For this review, take the finished solid that the model builds, in its own axes (mm). A direction names the side the tool comes from. Round coordinates to 2 decimals unless told otherwise and drop trailing zeros. Loops run counter-clockwise (first coordinate to the right, second up) from the corner with the lowest first, then second, coordinate; pieces in that order, holes last.
1) Mouldability with a two-part tool opening along Y and no side actions: class faces 4 (the cylindrical face through (-1.216, 1.115, 1.479)), 5 (the flat face through (34, 47, 1)), 6 (the flat face through (5.5, 44, 2)) as pulls with the +Y half, pulls with the -Y half, needs draft (parallel to the pull), parting line crosses it, or undercut.
2) Insertion check: pin 1 (19.5 mm diameter, centred on x = 10, z = 19, fed in from -Y); pin 2 (1 mm diameter, centred on x = 30, y = 7, fed in from +Z); pin 3 (3.5 mm diameter, centred on x = 21, z = 2, fed in from +Y); pin 4 (2.5 mm diameter, centred on x = 1, z = 10, fed in from +Y). Each pin has a flat end and moves straight along its axis. Give the tip position at first contact, or say it passes through.
3) Tool access review of faces 1 (the flat face through (17, 37, 14)), 2 (the cylindrical face through (30.07, 46.4, 1.48)), 3 (the flat face through (17, 34, 14)): name each direction out of +Z, -Z, +X, -X, +Y, -Y from which nothing blocks a thin tool from reaching the whole face with its end or side.
4) Take a section at B-B (z = 10). State the section outline as (x, y) points, then the cut area to 3 significant figures.
5) Take a section at D-D (y = 0). State the section outline as (x, z) points, then the cut area to 3 significant figures.
6) Take a section at A-A (y = 44). State the section outline as (x, z) points.
7) Take a section at C-C (x = 34). State the section outline as (y, z) points, then the cut area to 3 significant figures.
8) Wall thickness on L1, parallel to Z at x = 34, y = 35; L2, parallel to X at y = 34.75, z = 10; L3, parallel to Y at x = 0, z = 2.25: over which ranges is each line inside the solid? List them lowest first.
```python
from build123d import *

# Parameters (mm, degrees)
SKETCH1_W           = 41
SKETCH1_H           = 50
SKETCH1_R           = 1.65
BOSS_EXTRUDE1_DEPTH = 3
SKETCH2_W           = 41
SKETCH2_H           = 3
BOSS_EXTRUDE2_DEPTH = 30
SKETCH3_R           = 1.65
SKETCH3_R_2         = 7.5
CUT_EXTRUDE1_DEPTH  = 35
SKETCH4_W           = 24
SKETCH4_H           = 6
CUT_EXTRUDE2_DEPTH  = 10
FILLET2_R           = 2


with BuildPart() as part:
    # Sketch1 → Boss-Extrude1 (new body)
    with BuildSketch(Plane.XY):
        with Locations((17.5, 22)):
            Rectangle(SKETCH1_W, SKETCH1_H)
        with Locations((0, 44)):
            Circle(SKETCH1_R, mode=Mode.SUBTRACT)
        with Locations((35, 44)):
            Circle(SKETCH1_R, mode=Mode.SUBTRACT)
        with Locations((35, 0)):
            Circle(SKETCH1_R, mode=Mode.SUBTRACT)
        Circle(SKETCH1_R, mode=Mode.SUBTRACT)
    extrude(amount=BOSS_EXTRUDE1_DEPTH)

    # Sketch2 → Boss-Extrude2 (add)
    with BuildSketch(Plane.XY.offset(3)):
        with Locations((17.5, 35.5)):
            Rectangle(SKETCH2_W, SKETCH2_H)
    extrude(amount=BOSS_EXTRUDE2_DEPTH)

    # Sketch3 → Cut-Extrude1 (cut)
    with BuildSketch(Plane(origin=(0, 37, 0), x_dir=(1, 0, 0), z_dir=(0, 1, 0))):
        with Locations((34, -28)):
            Circle(SKETCH3_R)
        with Locations((34, -10)):
            Circle(SKETCH3_R)
        with Locations((1, -10)):
            Circle(SKETCH3_R)
        with Locations((1, -28)):
            Circle(SKETCH3_R)
        with Locations((10, -19)):
            Circle(SKETCH3_R_2)
    extrude(amount=-CUT_EXTRUDE1_DEPTH, mode=Mode.SUBTRACT)

    # Sketch4 → Cut-Extrude2 (cut)
    with BuildSketch(Plane.XY.offset(3)):
        with Locations((17.5, 44)):
            Rectangle(SKETCH4_W, SKETCH4_H)
    extrude(amount=-CUT_EXTRUDE2_DEPTH, mode=Mode.SUBTRACT)

    # Fillet2
    fillet2_edges = [part.edges().sort_by_distance(p)[0] for p in [
        (-3, 35.5, 33),
        (38, 35.5, 33),
        (5.5, 47, 1.5),
        (29.5, 47, 1.5),
        (-3, 47, 1.5),
        (38, 47, 1.5),
        (29.5, 41, 1.5),
        (5.5, 41, 1.5),
        (38, -3, 1.5),
        (-3, -3, 1.5),
    ]]
    fillet(fillet2_edges, radius=FILLET2_R)


solid = part.part
```
Response:
1. face 4: undercut
1. face 5: pulls with the +Y half
1. face 6: needs draft
2. pin 1: stops at y = 34
2. pin 2: stops at z = 3
2. pin 3: stops at y = 41
2. pin 4: passes through
3. face 1: +Z, +X, -X, +Y
3. face 2: +Z, -Z, +Y
3. face 3: +Z, +X, -X, -Y
4. outline: (-3, 34) - (-0.65, 34) - (-0.65, 37) - (-3, 37) - close; (2.65, 34) - (32.35, 34) - (32.35, 37) - (2.65, 37) - close; (35.65, 34) - (38, 34) - (38, 37) - (35.65, 37) - close
4. area: 103 mm2
5. outline: (-3, 0) - (-1.65, 0) - (-1.65, 3) - (-3, 3) - close; (1.65, 0) - (33.35, 0) - (33.35, 3) - (1.65, 3) - close; (36.65, 0) - (38, 0) - (38, 3) - (36.65, 3) - close
5. area: 103 mm2
6. outline: (-3, 0) - (-1.65, 0) - (-1.65, 3) - (-3, 3) - close; (1.65, 0) - (5.5, 0) - (5.5, 3) - (1.65, 3) - close; (29.5, 0) - (33.35, 0) - (33.35, 3) - (29.5, 3) - close; (36.65, 0) - (38, 0) - (38, 3) - (36.65, 3) - close
7. outline: (-3, 0) - (-1.31, 0) - (-1.31, 3) - (-3, 3) - close; (1.31, 0) - (42.69, 0) - (42.69, 3) - (37, 3) - (37, 8.35) - (34, 8.35) - (34, 3) - (1.31, 3) - close; (34, 11.65) - (37, 11.65) - (37, 26.35) - (34, 26.35) - close; (34, 29.65) - (37, 29.65) - (37, 33) - (34, 33) - close; (45.31, 0) - (47, 0) - (47, 3) - (45.31, 3) - close
7. area: 204 mm2
8. L1: z = 0 to 8.35, 11.65 to 26.35, 29.65 to 33
8. L2: x = -3 to -0.65, 2.65 to 32.35, 35.65 to 38
8. L3: y = -3 to -1.65, 1.65 to 42.35, 45.65 to 47
